Part print with two shaded views. Sizes in mm from the minimum x, y, z corner. Round coordinates to 2 decimals unless told otherwise and drop trailing zeros. Write each loop counter-clockwise with the first axis right and the second up, starting at its lowest first coordinate (ties: lowest second). Pieces come first, ordered by that corner, then holes. Notation, with made-up numbers: (59.5, -24) -> (89.5, -24) arc R23 ccw to (89.5, 10) -> close; hole circle Ø2 at (70, 89). An arc over 180 degrees is marked (long way). Return JSON: item names as keys, results as strings. Group by question number.
(1) Drill centre lines: L1, parallel to Y at x = 98, z = 0.9; L2, parallel to X at y = 6.5, z = 1.65; L3, parallel to X at y = 4, z = 0.2. Where is each one in solid material? Low to high. Write a range as from..to.
(2) Saw through at C-C (z = 0.6). List the corners of the cut face in (x, y), plus the area to 3 significant figures.
(3) Saw through at B-B (x = 36). List the corners of the cut face in (y, z).
(4) Saw through at A-A (y = 5). List the corners of the cut face in (x, z), plus the area to 3 significant figures.
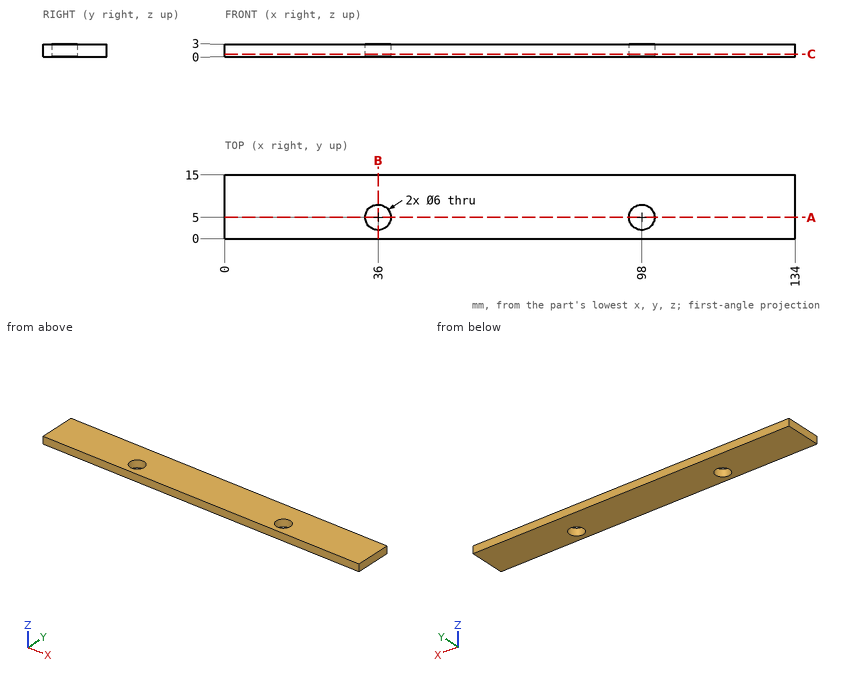
Computed values:
{
 "1": {"L1": "0..2, 8..15", "L2": "0..33.4, 38.6..95.4, 100.6..134", "L3": "0..33.17, 38.83..95.17, 100.83..134"},
 "2": {"outline": "(0, 0) -> (134, 0) -> (134, 15) -> (0, 15) -> close; hole circle Ø6 at (36, 5); hole circle Ø6 at (98, 5)", "area": "1,950 mm2"},
 "3": {"outline": "(0, 0) -> (2, 0) -> (2, 3) -> (0, 3) -> close; (8, 0) -> (15, 0) -> (15, 3) -> (8, 3) -> close"},
 "4": {"outline": "(0, 0) -> (33, 0) -> (33, 3) -> (0, 3) -> close; (39, 0) -> (95, 0) -> (95, 3) -> (39, 3) -> close; (101, 0) -> (134, 0) -> (134, 3) -> (101, 3) -> close", "area": "366 mm2"}
}
